The listing builds one solid part. Answer for the finished solid, in the listing's coordinates (mm). Coordinates: 2 decimals unless noted, no trailing zeros. Loops run counter-clockwise (first coordinate to the right, second up) from the corner with the lowest first, then second, coordinate; pieces in that order, holes last. Notation, with made-up numbers: (-18.75, -28) - (-0.75, -28) arc R32 cw to (-0.75, 5) - close; hole circle Ø7 at (75, 34). An arc over 180 degrees is marked (long way). Return JSON: item names as keys, results as strings. Group by question number.
1. Each of these flat-tipped pins is pushed along its axis until it touches: P1, Ø3, axis at x = -3.5, y = -87.5, coming from the +Z side; P2, Ø0.6, axis at y = -201.5, z = -2.5, coming from the -X side; P3, Ø0.6, axis at y = -253, z = -2.5, coming from the +X side; P4, Ø2.5, axis at x = 0, y = -15, coming from the -Z side. Where does it stop, or does it pass through?
2. Find the intervals of material crossed by line 1 along X through (y, z) = (-327, -1.05); line 2 along X through (y, z) = (-27, 1.8); line 3 along Z through (x, y) = (7, -32), in increasing order.
3. Section A-A (y = -293) is taken. Write down the section's boundary in (x, z), and give its area (3 significant figures).
```python
from build123d import *

# Parameters (mm, degrees)
F1_DEPTH = 400
F2_R     = 1.6
F3_DEPTH = 25


with BuildPart() as f1:
    # F0 (on Front) → F1 (new body)
    with BuildSketch(Plane.XZ):
        Polygon((6, 0), (0, 0), (-6, 0), (-6, 2), (-9, 2), (-9, -2), (-4, -2), (-4, -2.5), (0, -2.5), (4, -2.5), (4, -2), (9, -2), (9, 2), (6, 2), align=None)
    extrude(amount=F1_DEPTH)

    # F2 (on face) → F3 (cut)
    with BuildSketch(Plane.XY):
        with Locations((0, -15)):
            Circle(F2_R)
        with Locations((0, -54)):
            Circle(F2_R)
        with Locations((0, -93)):
            Circle(F2_R)
        with Locations((0, -132)):
            Circle(F2_R)
        with Locations((0, -171)):
            Circle(F2_R)
        with Locations((0, -210)):
            Circle(F2_R)
        with Locations((0, -249)):
            Circle(F2_R)
        with Locations((0, -288)):
            Circle(F2_R)
        with Locations((0, -327)):
            Circle(F2_R)
        with Locations((0, -366)):
            Circle(F2_R)
    extrude(amount=-F3_DEPTH, mode=Mode.SUBTRACT)


solid = f1.part
```
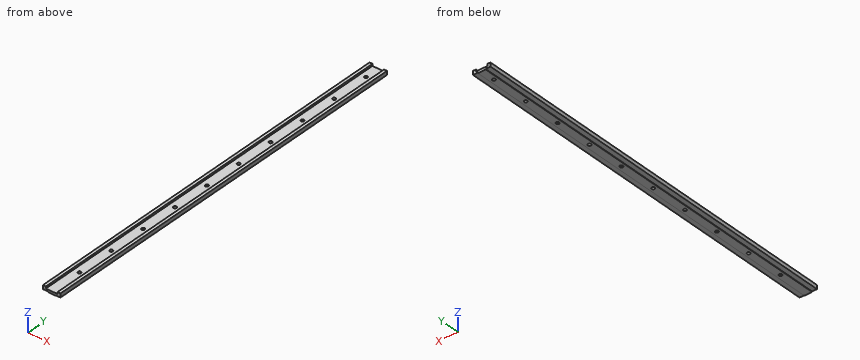
The answers:
{
 "1": {"P1": "stops at z = 0", "P2": "stops at x = -4", "P3": "stops at x = 4", "P4": "passes through"},
 "2": {"line 1": "x = -9 to -1.6, 1.6 to 9", "line 2": "x = -9 to -6, 6 to 9", "line 3": "z = -2 to 2"},
 "3": {"outline": "(-9, -2) - (-4, -2) - (-4, -2.5) - (4, -2.5) - (4, -2) - (9, -2) - (9, 2) - (6, 2) - (6, 0) - (-6, 0) - (-6, 2) - (-9, 2) - close", "area": "52.0 mm2"}
}
